Input: part model. Units: mm. Frame: model coordinates. A direction names the side the tool comes from. Give positions to 0.01 mm unless a question says otherwise; leave off trailing zeros. Loops run counter-clockwise (first coordinate to the right, second up) from the corner with the lowest first, then second, coordinate; pieces in that order, holes last. Notation, with made-up numbers: (55, 10.5) -> (102, 10.5) arc R24 ccw to (102, 28.5) -> close; hole circle Ø9 at (24.25, 52). An arc over 180 degrees is marked (long way). Answer as a JSON object with one key per item and string values.
```python
from build123d import *

# Parameters (mm, degrees)
F0_W     = 100
F0_H     = 300
F1_DEPTH = 2
F2_W     = 100
F2_H     = 200
F3_DEPTH = 10
F4_W     = 100
F4_H     = 100
F5_DEPTH = 25
F6_R     = 10
F7_R     = 4
F8_DEPTH = 37.001
F9_SIZE  = 1.5


# Not quite as in the source:
# - a pattern or mirror of a feature is missing from the dataset's text; its kind, count and spacing are read off the source's solid


with BuildPart() as f1:
    # F0 (on Top) → F1 (new body)
    with BuildSketch(Plane.XY):
        Rectangle(F0_W, F0_H)
    extrude(amount=F1_DEPTH)

    # F2 (on face) → F3 (join)
    with BuildSketch(Plane.XY.offset(2)):
        with Locations((0, 50)):
            Rectangle(F2_W, F2_H)
    extrude(amount=F3_DEPTH)

    # F4 (on face) → F5 (join)
    with BuildSketch(Plane.XY.offset(12)):
        with Locations((0, 100)):
            Rectangle(F4_W, F4_H)
    extrude(amount=F5_DEPTH)

    # F6
    f6_edges = [f1.edges().sort_by_distance(p)[0] for p in [
        (-50, 150, 18.5),
        (-50, -150, 1),
        (50, -150, 1),
        (50, 150, 18.5),
    ]]
    fillet(f6_edges, radius=F6_R)

    # F7 (on face) → F8 (cut, through all)
    with BuildSketch(Plane.XY.offset(37)):
        with Locations((-40, 140)):
            Circle(F7_R)
    f8 = extrude(amount=-F8_DEPTH, mode=Mode.SUBTRACT)

    # F8_copies: F8 across plane
    add(f8.mirror(Plane(origin=(0, 0, 0), x_dir=(0, 0, 1), z_dir=(1, 0, 0))), mode=Mode.SUBTRACT)

    # F9
    f9_edges = [f1.edges().sort_by_distance(p)[0] for p in [
        (-44, 140, 37),
        (-36, 140, 18.5),
        (-44, 140, 0),
        (44, 140, 0),
        (44, 140, 37),
    ]]
    chamfer(f9_edges, length=F9_SIZE)


solid = f1.part
```
Q1. Section D-D, the plane z = 20.5. Return the cut outline in (x, y).
Evaluation:
{"outline": "(-50, 50) -> (50, 50) -> (50, 140) arc R10 ccw to (40, 150) -> (-40, 150) arc R10 ccw to (-50, 140) -> close; hole circle Ø8 at (-40, 140); hole circle Ø8 at (40, 140)"}
Q2. Section B-B, the plane z = 5. Return the cut outline in (x, y), then the cut area to 3 significant figures.
Evaluation:
{"outline": "(-50, -50) -> (50, -50) -> (50, 140) arc R10 ccw to (40, 150) -> (-40, 150) arc R10 ccw to (-50, 140) -> close; hole circle Ø8 at (-40, 140); hole circle Ø8 at (40, 140)", "area": "19,900 mm2"}
Q3. Section A-A, the plane x = -13. Return the cut outline in (y, z).
Evaluation:
{"outline": "(-150, 0) -> (150, 0) -> (150, 37) -> (50, 37) -> (50, 12) -> (-50, 12) -> (-50, 2) -> (-150, 2) -> close"}
Q4. Pin query (flat end, axial travel): pin 1 (10 mm diameter, centred on x = 25.5, y = -105, fed in from +Z); pin 2 (7.5 mm diameter, centred on x = 23.5, z = 26, fed in from -Y). Return the tip coordinate at first contact, or that it passes through.
Evaluation:
{"pin 1": "stops at z = 2", "pin 2": "stops at y = 50"}
Q5. Access query for faces 1 (the cylindrical face through (47.15, -146.99, 1.01)), 2 (the flat face through (-1, 50, 24)). Directions: +Z, -Z, +X, -X, +Y, -Y. A direction counts if a zero-diameter tool reaches every point of the face in a straight line with its end or side. Return the directions, or none.
Evaluation:
{"face 1": "+Z, -Z, +X, -Y", "face 2": "+Z, +X, -X, -Y"}
Q6. Ray query, line 1 along Y through (x, z) = (40.5, 22.5); line 2 along Y through (x, z) = (40, 9); line 3 along Z through (x, y) = (-19.5, -44.5). Return the intervals inside material, ascending.
Evaluation:
{"line 1": "y = 50 to 136.03, 143.97 to 149.99", "line 2": "y = -50 to 136, 144 to 150", "line 3": "z = 0 to 12"}
Q7. Section C-C, the plane y = -93.5. Return the cut outline in (x, z).
Evaluation:
{"outline": "(-50, 0) -> (50, 0) -> (50, 2) -> (-50, 2) -> close"}
Q8. Draft query along Y for faces 3 (the cylindrical face through (40.521, 143.966, 18.738)), 4 (the flat face through (-1, 150, 18)), 5 (the flat face through (-50, 60, 14)). Return one class per face: +Y half, -Y half, draft (parallel to the pull), parting line (faces both ways), or undercut.
Evaluation:
{"face 3": "undercut", "face 4": "+Y half", "face 5": "draft"}
